For this review, take the finished solid that the model builds, in its own axes (mm). Round coordinates to 2 decimals unless told otherwise and drop trailing zeros. Loops run counter-clockwise (first coordinate to the right, second up) from the corner with the lowest first, then second, coordinate; pieces in that order, holes last.
1. Consider section C-C on x = -58. State the section outline as (y, z) points.
2. To check wall thickness, follow line 1 along X through (y, z) = (0, 0.35); line 2 along X through (y, z) = (-7, -0.2); line 3 along Y through (x, z) = (6.5, 0.05). State the ranges of each line that lie inside material, in increasing order.
3. Clearance check with flat-ended pins moving along their axes: pin 1 Ø1.5 at (y, z) = (-10.5, -1.5) entering from -X; pin 2 Ø1 at (y, z) = (9, -0.5) entering from +X; pin 3 Ø14.5 at (x, y) = (-49.6, 0) entering from +Z. State where each tip first meets the part, or that it passes through.
4. Consider section D-D on x = 16. State the section outline as (y, z) points.
5. Consider section B-B on z = 0. State the section outline as (x, y) points.
6. Consider section A-A on y = 0. State the section outline as (x, z) points, then the cut area to 3 significant figures.
Autodesk Inventor part; units mm, degrees
ref_plane "YZ Plane" through (0, 0, 0) normal (1, 0, 0) x (0, 1, 0)
ref_plane "XZ Plane" through (0, 0, 0) normal (0, 1, 0) x (-1, 0, 0)
ref_plane "XY Plane" through (0, 0, 0) normal (0, 0, 1) x (1, 0, 0)
sketch "Sketch1" plane through (0, 0, 0) normal (1, 0, 0) x (0, 1, 0)
  circle A0 centre (0, 0) radius 2.5
  dimension "d0" = 5
extrude "Extrusion1" add sketch "Sketch1" along normal mid plane 80
sketch "Sketch3" plane through (0, 0, 0) normal (0, 0, 1) x (1, 0, 0)
  circle A0 centre (-49.5974, 0) radius 12
  circle A1 centre (-49.5974, 0) radius 14
  point P0 (0, 0)
  dimension "d6" = 24
  dimension "d7" = 28
extrude "Extrusion3" add sketch "Sketch3" along normal mid plane 2
sketch "Sketch4" plane through (40, 0, 0) normal (1, 0, 0) x (0, 0, -1)
  circle A0 centre (0, 0) radius 2.5
extrude "Extrusion4" cut sketch "Sketch4" against normal blind 10
properties part number "SS-5FL111-3T_Housing_02"
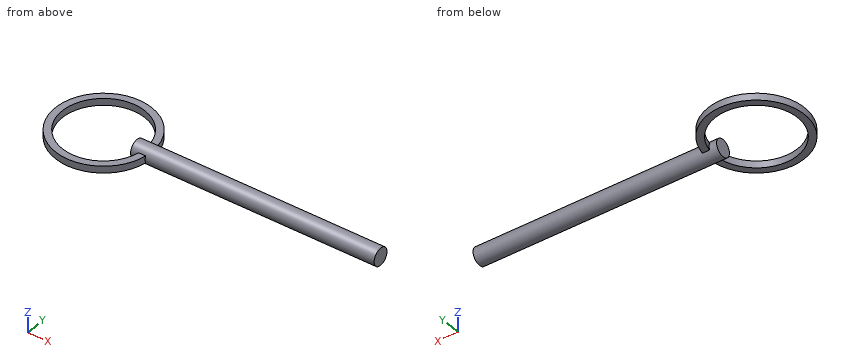
Resolved:
1. outline: (-11.2, -1) - (-8.57, -1) - (-8.57, 1) - (-11.2, 1) - close; (8.57, -1) - (11.2, -1) - (11.2, 1) - (8.57, 1) - close
2. line 1: x = -63.6 to -61.6, -40 to 30
2. line 2: x = -61.72 to -59.34, -39.85 to -37.47
2. line 3: y = -2.5 to 2.5
3. pin 1: stops at x = -59.46
3. pin 2: stops at x = -38.47
3. pin 3: passes through
4. outline: circle Ø5 at (0, 0)
5. outline: (-35.82, -2.5) - (30, -2.5) - (30, 2.5) - (-35.82, 2.5) arc R14 ccw (long way) to start; hole (-40, -2.5) - (-40, 2.5) - (-37.86, 2.5) arc R12 ccw (long way) to (-37.86, -2.5) - close
6. outline: (-63.6, -1) - (-61.6, -1) - (-61.6, 1) - (-63.6, 1) - close; (-40, -2.5) - (30, -2.5) - (30, 2.5) - (-40, 2.5) - close
6. area: 354 mm2
